from build123d import *

# Parameters (mm, degrees)
BOSS_EXTRUDE1_DEPTH = 1.5
FILLET1_R           = 1
SKETCH5_R           = 2.5
BOSS_EXTRUDE2_DEPTH = 8


with BuildPart() as part:
    # Sketch1 → Boss-Extrude1 (new body)
    with BuildSketch(Plane(origin=(0, 0, 0), x_dir=(1, 0, 0), z_dir=(0, 1, 0))):
        with BuildLine():
            Line((-13, -19), (13, -19))
            ThreePointArc((13, -19), (17.242640687, -17.242640687), (19, -13))
            Line((19, -13), (19, 13))
            ThreePointArc((19, 13), (17.242640687, 17.242640687), (13, 19))
            Line((13, 19), (-13, 19))
            ThreePointArc((-13, 19), (-17.242640687, 17.242640687), (-19, 13))
            Line((-19, 13), (-19, -13))
            ThreePointArc((-19, -13), (-17.242640687, -17.242640687), (-13, -19))
        make_face()
        with BuildLine():
            Line((-12.61109127, 16.570889245), (-9.429110755, 13.38890873))
            ThreePointArc((-9.429110755, 13.38890873), (-9.429110755, 9.429110755), (-13.38890873, 9.429110755))
            Line((-13.38890873, 9.429110755), (-16.570889245, 12.61109127))
            ThreePointArc((-16.570889245, 12.61109127), (-16.570889245, 16.570889245), (-12.61109127, 16.570889245))
        make_face(mode=Mode.SUBTRACT)
        with BuildLine():
            Line((16.570889245, 12.61109127), (13.38890873, 9.429110755))
            ThreePointArc((13.38890873, 9.429110755), (9.429110755, 9.429110755), (9.429110755, 13.38890873))
            Line((9.429110755, 13.38890873), (12.61109127, 16.570889245))
            ThreePointArc((12.61109127, 16.570889245), (16.570889245, 16.570889245), (16.570889245, 12.61109127))
        make_face(mode=Mode.SUBTRACT)
        with BuildLine():
            Line((12.61109127, -16.570889245), (9.429110755, -13.38890873))
            ThreePointArc((9.429110755, -13.38890873), (9.429110755, -9.429110755), (13.38890873, -9.429110755))
            Line((13.38890873, -9.429110755), (16.570889245, -12.61109127))
            ThreePointArc((16.570889245, -12.61109127), (16.570889245, -16.570889245), (12.61109127, -16.570889245))
        make_face(mode=Mode.SUBTRACT)
        with BuildLine():
            Line((-16.570889245, -12.61109127), (-13.38890873, -9.429110755))
            ThreePointArc((-13.38890873, -9.429110755), (-9.429110755, -9.429110755), (-9.429110755, -13.38890873))
            Line((-9.429110755, -13.38890873), (-12.61109127, -16.570889245))
            ThreePointArc((-12.61109127, -16.570889245), (-16.570889245, -16.570889245), (-16.570889245, -12.61109127))
        make_face(mode=Mode.SUBTRACT)
    extrude(amount=BOSS_EXTRUDE1_DEPTH)

    # Sketch3 → Revolve1 (revolve)
    with BuildSketch(Plane(origin=(0, 0, 0), x_dir=(0, 0, -1), z_dir=(1, 0, 0))):
        Polygon((0, 1.5), (13, 1.5), (10, 4.5), (0, 4.5), align=None)
    revolve(axis=Axis((0, 4.5, 0), (0, -1, 0)))

    # Sketch4 → Cut-Revolve1 (revolve, cut)
    with BuildSketch(Plane(origin=(0, 0, 0), x_dir=(0, 0, -1), z_dir=(1, 0, 0)), mode=Mode.PRIVATE) as cut_revolve1_sk:
        Polygon((0, 0), (12, 0), (8, 4), (0, 4), align=None)
    revolve(cut_revolve1_sk.sketch.rotate(Axis((0, 4, 0), (0, -1, 0)), 180), axis=Axis((0, 4, 0), (0, -1, 0)), mode=Mode.SUBTRACT)

    # Fillet1
    fillet1_edges = [part.edges().sort_by_distance(p)[0] for p in [
        (0, 0, -12),
        (0, 4, -8),
    ]]
    fillet(fillet1_edges, radius=FILLET1_R)

    # Sketch5 → Boss-Extrude2 (add)
    with BuildSketch(Plane(origin=(0, 4.5, 0), x_dir=(1, 0, 0), z_dir=(0, 1, 0))):
        with Locations(Location((0, 0, 0), (0, 0, 90))):
            Circle(SKETCH5_R)
    extrude(amount=BOSS_EXTRUDE2_DEPTH)


solid = part.part
CAD build for the part. Positions are in the model's coordinates, mm. A direction names the side the tool comes from. Round coordinates to 2 decimals unless told otherwise and drop trailing zeros. Write each loop counter-clockwise with the first axis right and the second up, starting at its lowest first coordinate (ties: lowest second). Pieces come first, ordered by that corner, then holes. Notation, with made-up numbers: (45, 85.25) -> (96, 85.25) arc R32 cw to (96, 112.25) -> close; hole circle Ø1 at (20, 61.5). An arc over 180 degrees is marked (long way). Answer as a JSON object with one key per item and string values.
(1) Probe probe 1 along Z at (x, y) = (12, 0.75); probe 2 along Y at (x, z) = (3, -4); probe 3 along Z at (x, y) = (7.5, 1.25). List the from-to ranges inside material, lowest first. Write a range as [from, to].
Reported:
{"probe 1": "z = [-19, -15.96], [-8.67, 8.67], [15.96, 19]", "probe 2": "y = [4, 4.5]", "probe 3": "z = [-19, -7.7], [7.7, 19]"}
(2) Band-saw the part on D-D, the plane y = 2.75. List the corners of the cut face in (x, z).
Reported:
{"outline": "circle Ø23.5 at (0, 0); hole circle Ø18.5 at (0, 0)"}
(3) Band-saw the part on B-B, the plane x = 0. List the corners of the cut face in (y, z).
Reported:
{"outline": "(0, -19) -> (1.5, -19) -> (1.5, -13) -> (4.5, -10) -> (4.5, -2.5) -> (12.5, -2.5) -> (12.5, 2.5) -> (4.5, 2.5) -> (4.5, 10) -> (1.5, 13) -> (1.5, 19) -> (0, 19) -> (0, 12.41) arc R1 ccw to (0.29, 11.71) -> (3.71, 8.29) arc R1 cw to (4, 7.59) -> (4, -7.59) arc R1 cw to (3.71, -8.29) -> (0.29, -11.71) arc R1 ccw to (0, -12.41) -> close"}
(4) Which spindle directions (+Z, -Z, +X, -X, +Y, -Y) get a long thin tool onto all of the face, cutting with end or side? Do faces 1 (the face through (-2, 4.5, -2)), 2 (the face through (-19, 1, 0)), 3 (the face through (-11, 0.74, 14.96)). Say none if no direction does.
Reported:
{"face 1": "+Y", "face 2": "+Z, -Z, -X, +Y, -Y", "face 3": "+Y, -Y"}
(5) Band-saw the part on C-C, the plane z = 0. List the corners of the cut face in (x, y).
Reported:
{"outline": "(-19, 0) -> (-12.41, 0) arc R1 ccw to (-11.71, 0.29) -> (-8.29, 3.71) arc R1 cw to (-7.59, 4) -> (7.59, 4) arc R1 cw to (8.29, 3.71) -> (11.71, 0.29) arc R1 ccw to (12.41, 0) -> (19, 0) -> (19, 1.5) -> (13, 1.5) -> (10, 4.5) -> (2.5, 4.5) -> (2.5, 12.5) -> (-2.5, 12.5) -> (-2.5, 4.5) -> (-10, 4.5) -> (-13, 1.5) -> (-19, 1.5) -> close"}
(6) Two-plate mould, pull along X, no slides. Class faces 4 (the face through (9.47, 0.74, -9.39)), 5 (the face through (17.289, 0.74, -17.196)), 6 (the face through (-17.196, 0.74, -17.289)): +X half, -X half, draft (parallel to the pull), parting line (faces both ways), or undercut.
Reported:
{"face 4": "undercut", "face 5": "+X half", "face 6": "-X half"}
(7) Band-saw the part on A-A, the plane x = -15. List the corners of the cut face in (y, z), then the cut area to 3 significant figures.
Reported:
{"outline": "(0, -18.66) -> (1.5, -18.66) -> (1.5, -17.36) -> (0, -17.36) -> close; (0, -11.04) -> (1.5, -11.04) -> (1.5, 11.04) -> (0, 11.04) -> close; (0, 17.36) -> (1.5, 17.36) -> (1.5, 18.66) -> (0, 18.66) -> close", "area": "37.0 mm^2"}
(8) Pin check, flat tips, straight feed: P1, Ø16.5, axis at x = -3.5, z = 0.5, coming from the -Y side; P2, Ø10, axis at x = 3, z = -1.5, coming from the -Y side. Stop position of each tip, or through.
Reported:
{"P1": "stops at y = 0.22", "P2": "stops at y = 3.65"}
